```python
from build123d import *

# Parameters (mm, degrees)
PAD001_DEPTH    = 25
SKETCH002_R     = 1.1
POCKET_DEPTH    = 20.276252
POCKET002_DEPTH = 40.001
SKETCH_R        = 12
PAD_DEPTH       = 5
SKETCH003_R     = 1.1
POCKET001_DEPTH = 50.001


with BuildPart() as f_10degcut:
    # Sketch001 → Pad001 (new body)
    with BuildSketch(Plane(origin=(0, -0.3, 2.2), x_dir=(1, 0, 0), z_dir=(0, 0.173648, 0.984808))):
        with BuildLine():
            Line((-15.716234, -3), (-20, -3))
            Line((-20, -3), (-20, 0))
            Line((-20, 0), (-14, 0))
            ThreePointArc((-14, 0), (0, -14), (14, 0))
            Line((14, 0), (20, 0))
            Line((20, 0), (20, -3))
            Line((20, -3), (15.716234, -3))
            ThreePointArc((-15.716234, -3), (0, -16), (15.716234, -3))
        make_face()
    extrude(amount=PAD001_DEPTH)

    # Sketch002 → Pocket (cut, through all)
    with BuildSketch(Plane(origin=(0, -0.3, 2.2), x_dir=(-1, 0, 0), z_dir=(0, 0.984808, -0.173648))):
        with Locations((-17.5, 22)):
            Circle(SKETCH002_R)
        with Locations((-17.5, 12)):
            Circle(SKETCH002_R)
        with Locations((17.5, 22)):
            Circle(SKETCH002_R)
        with Locations((17.5, 12)):
            Circle(SKETCH002_R)
    extrude(amount=-POCKET_DEPTH, mode=Mode.SUBTRACT)

    # Sketch004 → Pocket002 (cut, through all)
    with BuildSketch(Plane(origin=(20, -0.3, 2.2), x_dir=(0, 0.984808, -0.173648), z_dir=(1, 0, 0))):
        Polygon((0, 0), (0, 2.821232), (-16, 0), align=None)
    extrude(amount=-POCKET002_DEPTH, mode=Mode.SUBTRACT)


with BuildPart() as fusion:
    # Sketch → Pad (new body)
    with BuildSketch(Plane.XY):
        with BuildLine():
            Line((-20, 25), (-20, -25))
            Line((-20, -25), (-15, -25))
            Line((-15, -25), (-15, -5.567764))
            ThreePointArc((-15, -5.567764), (0, -16), (15, -5.567764))
            Line((15, -25), (15, -5.567764))
            Line((20, -25), (15, -25))
            Line((20, 25), (20, -25))
            Line((15, 25), (20, 25))
            Line((15, 5.567764), (15, 25))
            ThreePointArc((15, 5.567764), (0, 16), (-15, 5.567764))
            Line((-15, 25), (-15, 5.567764))
            Line((-20, 25), (-15, 25))
        make_face()
        Circle(SKETCH_R, mode=Mode.SUBTRACT)
    extrude(amount=PAD_DEPTH)

    # Sketch003 → Pocket001 (cut, through all)
    with BuildSketch(Plane(origin=(0, 25, 0), x_dir=(-1, 0, 0), z_dir=(0, 1, 0))):
        with Locations((-17.5, 2.5)):
            Circle(SKETCH003_R)
        with Locations((17.5, 2.5)):
            Circle(SKETCH003_R)
    extrude(amount=-POCKET001_DEPTH, mode=Mode.SUBTRACT)

    # Fusion: union 10degCut
    add(f_10degcut.part)


solid = fusion.part
```
Can you work these out from the model? Positions are in its coordinate system, mm. A direction names the side the tool comes from. Give positions to 0.01 mm unless a question says otherwise; leave off trailing zeros. Order: outer loops, then holes, each group sorted by start corner. A loop starts at its lowest first (then second) coordinate and runs counter-clockwise, first axis right, second up. Notation, with made-up numbers: M 88,-8.75 L 136,-8.75 A26 ccw 136,16.25 Z; hole C -27,30 d6. An arc over 180 degrees is marked long. One line per item, written item: value.
1) Please list where these lines run through material, in increasing order: line 1 along Y through (x, z) = (0, 1.3); line 2 along Z through (x, y) = (17.5, 15); line 3 along X through (y, z) = (-3.5, 2.75).
Answer sheet:
line 1: y = -16 to -12, 12 to 16
line 2: z = 0 to 1.4, 3.6 to 5
line 3: x = -20 to -18.57, -16.43 to -11.48, 11.48 to 16.43, 18.57 to 20
2) I want a section at A-A, the plane y = -18.5. List the corners of the cut face in (x, z) for me.
Answer sheet:
outline: M -20,0 L -15,0 L -15,5 L -20,5 Z; M 15,0 L 20,0 L 20,5 L 15,5 Z; hole C -17.5,2.5 d2.2; hole C 17.5,2.5 d2.2
3) I want a section at D-D, the plane x = 17.5. List the corners of the cut face in (y, z) for me, plus the area to 3 significant figures.
Answer sheet:
outline: M -25,0 L 25,0 L 25,1.4 L -25,1.4 Z; M -25,3.6 L 25,3.6 L 25,5 L 0.19,5 L 1.59,12.93 L -1.36,13.46 L -2.85,5 L -25,5 Z; M -0.98,15.62 L 1.97,15.1 L 3.33,22.78 L 0.37,23.3 Z; M 0.76,25.47 L 3.71,24.95 L 4.04,26.82 L 1.09,27.34 Z
area: 194 mm^2
4) We'd pull the mould along X, two halves only. Please class faces 4 (the face through (-17, -14, 5)), 5 (the face through (-20, 0, 4)), 6 (the face through (18.37, 1.95, 23.46)): released by +X, released by -X, zero draft, split by the parting line, or undercut.
Answer sheet:
face 4: zero draft
face 5: released by -X
face 6: undercut
5) I want a section at B-B, the plane y = 9. List the corners of the cut face in (x, z) for me, plus the area to 3 significant figures.
Answer sheet:
outline: M -20,0 L -15,0 L -15,5 L -20,5 Z; M -13.23,0 L -7.94,0 L -7.94,5 L -13.23,5 Z; M 7.94,0 L 13.23,0 L 13.23,5 L 7.94,5 Z; M 15,0 L 20,0 L 20,5 L 15,5 Z; hole C -17.5,2.5 d2.2; hole C 17.5,2.5 d2.2
area: 95.3 mm^2
6) For P1, Ø5, axis at x = 13.5, z = 12.5, coming from the +Y side; P2, Ø8, axis at y = -12, z = 17, coming from the -X side; P3, Ø8, axis at x = 17, y = -12, coming from the +Z side, each with a flat end and sliding along its axis, tell me the tip position at first contact or that it passes through.
Answer sheet:
P1: stops at y = 1.95
P2: stops at x = -12.42
P3: stops at z = 5
7) On a 3-axis mill with a long thin cutter (end or side, diameter ignored), from which of +Z, -Z, +X, -X, +Y, -Y can I reach the whole of each face in a straight line? I mean faces 1 (the face through (-17, 2.1, 15.8)), 2 (the face through (-15, 15, 2)), 3 (the face through (18, -14, 5)). Say none if no direction works.
Answer sheet:
face 1: +X, -X, +Y
face 2: +Z, -Z, +Y
face 3: +Z, +X, -Y
8) I want a section at C-C, the plane x = 4.5. List the corners of the cut face in (y, z) for me.
Answer sheet:
outline: M -15.4,4.98 L -15.35,4.98 L -15.35,0 L -11.12,0 L -11.12,5 L -13.27,5 L -9.01,29.12 L -11.08,29.49 Z; M 11.12,0 L 15.35,0 L 15.35,5 L 11.12,5 Z
